```python
from build123d import *

# Parameters (mm, degrees)
SKETCH_1_W      = 1800
SKETCH_1_H      = 2100
EXTRUDE_1_DEPTH = 250
SKETCH_2_W      = 586.997926232
SKETCH_2_H      = 343.897774964
EXTRUDE_2_DEPTH = 158


with BuildPart() as part:
    # Эскиз1 → Бобышка-Вытянуть1 (new, symmetric)
    with BuildSketch(Plane(origin=(0, 0, 0), x_dir=(1, 0, 0), z_dir=(0, 1, 0))):
        with Locations((900, 1050)):
            Rectangle(SKETCH_1_W, SKETCH_1_H)
    extrude(amount=EXTRUDE_1_DEPTH, both=True)

    # Эскиз2 → Бобышка-Вытянуть2 (add)
    with BuildSketch(Plane(origin=(0, 250, 0), x_dir=(1, 0, 0), z_dir=(0, 1, 0))):
        with Locations((490.880233232, 1829.277683609)):
            Rectangle(SKETCH_2_W, SKETCH_2_H)
        with Locations((1288.36731483, 1829.277683609)):
            Rectangle(SKETCH_2_W, SKETCH_2_H)
    extrude(amount=EXTRUDE_2_DEPTH)


solid = part.part
```
Model file for the job. Use its own axes, mm. A direction names the side the tool comes from. Coordinates: 2 decimals unless noted, no trailing zeros. Write each loop counter-clockwise with the first axis right and the second up, starting at its lowest first coordinate (ties: lowest second). Pieces come first, ordered by that corner, then holes. Notation, with made-up numbers: (18, -15) - (76, -15) arc R8 ccw to (76, -9) - close; hole circle Ø10 at (24, 63.5). An arc over 180 degrees is marked (long way). One line per question, with ' | ' between items. Start each with the question number.
Q1. Pull direction X, two halves, no side cores. Call faces 5 (the face through (1581.866, 328, -1827)), 6 (the face through (784.379, 328, -1827)), 7 (the face through (197.381, 328, -1827)): pulls with the +X half, pulls with the -X half, needs draft (parallel to the pull), parting line crosses it, or undercut.
Q2. Cut at B-B, the plane z = -1930. List the corners of the cut face in (x, y).
Q3. Cut at D-D, the plane z = -1350. List the corners of the cut face in (x, y).
Q4. Drill centre lines: line 1 (X direction, y = 303, z = -1693.5); line 2 (Y direction, x = 181.5, z = -1533.5); line 3 (Z direction, x = 1326, y = 330.5). Where is each one in solid material? Low to high. Write a range as [from, to].
Q5. 3-axis set-ups, long thin cutter, end or side, ignore diameter. For faces 1 (the face through (1800, 4, -1035)), 2 (the face through (994.868, 328, -1827)), 3 (the face through (487, 328, -2001.227)), 4 (the face through (1284, 328, -1657.329)): which of +Z, -Z, +X, -X, +Y, -Y reach the whole face in a straight line?
Q6. Pin check, flat tips, straight feed: pin 1 (2 mm diameter, centred on x = 521.5, y = 272, fed in from -Z); pin 2 (1.5 mm diameter, centred on y = 297.5, z = -1795.5, fed in from -X). Stop position of each tip, or through.
Q7. Cut at A-A, the plane y = 300.5. List the corners of the cut face in (x, z), then the cut area to 3 significant figures.
Q8. Cut at C-C, the plane x = 353. List the corners of the cut face in (y, z), then the cut area to 3 significant figures.
Answer below:
1) face 5: pulls with the +X half | face 6: undercut | face 7: pulls with the -X half
2) outline: (0, -250) - (1800, -250) - (1800, 250) - (1581.87, 250) - (1581.87, 408) - (994.87, 408) - (994.87, 250) - (784.38, 250) - (784.38, 408) - (197.38, 408) - (197.38, 250) - (0, 250) - close
3) outline: (0, -250) - (1800, -250) - (1800, 250) - (0, 250) - close
4) line 1: [197.38, 784.38], [994.87, 1581.87] | line 2: [-250, 250] | line 3: [-2001.23, -1657.33]
5) face 1: +Z, -Z, +X, +Y, -Y | face 2: +Z, -Z, +Y | face 3: -Z, +X, -X, +Y | face 4: +Z, +X, -X, +Y
6) pin 1: z = -2001.23 | pin 2: x = 197.38
7) outline: (197.38, -2001.23) - (784.38, -2001.23) - (784.38, -1657.33) - (197.38, -1657.33) - close; (994.87, -2001.23) - (1581.87, -2001.23) - (1581.87, -1657.33) - (994.87, -1657.33) - close | area: 404,000 mm^2
8) outline: (-250, -2100) - (250, -2100) - (250, -2001.23) - (408, -2001.23) - (408, -1657.33) - (250, -1657.33) - (250, 0) - (-250, 0) - close | area: 1,100,000 mm^2
